Verification items for this drawing (mm, ordinates from the low corner). A direction names the side the tool comes from. Coordinates: 2 decimals unless noted, no trailing zeros. Order: outer loops, then holes, each group sorted by start corner. A loop starts at its lowest first (then second) coordinate and runs counter-clockwise, first axis right, second up. Notation, with made-up numbers: (-14, -26) - (30, -26) arc R25 cw to (30, -14) - close; hole circle Ø1 at (17, -10.5). An arc over 180 degrees is marked (long way). One line per question, with ' | ' between items. Start each with the question number.
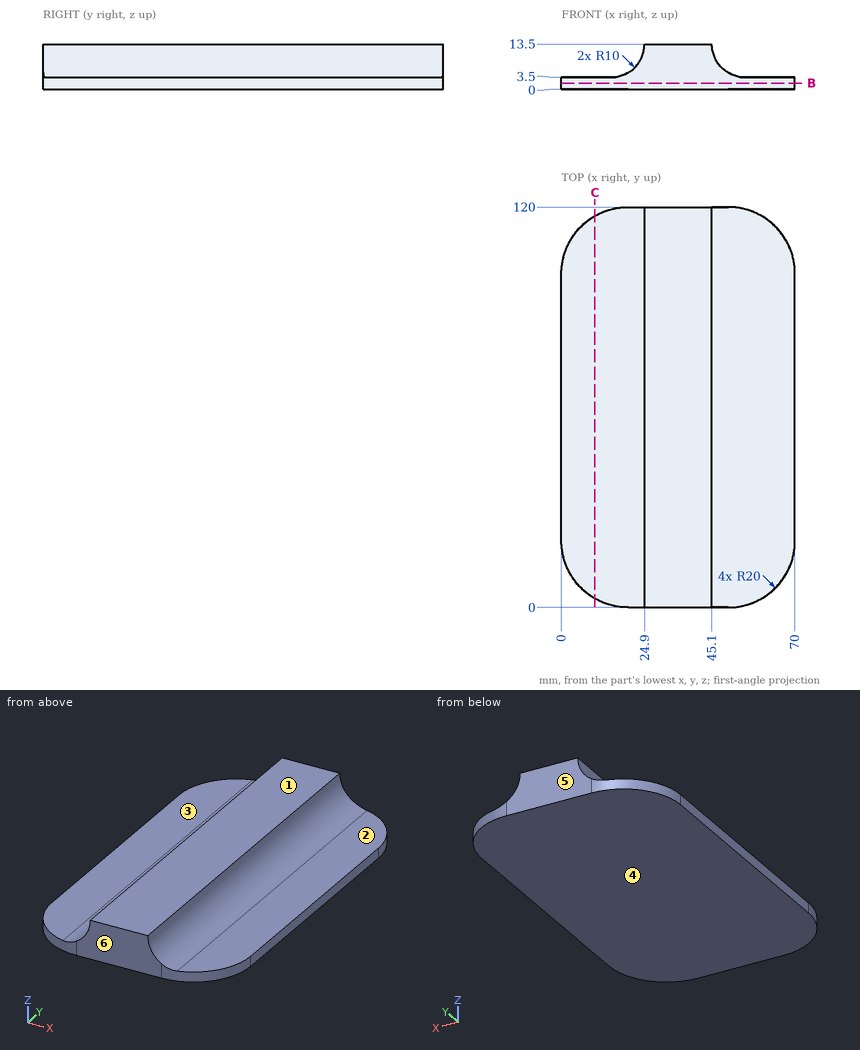
Item 1: Section check B-B (z = 1.75). Record the cut outline in (x, y).
Item 2: Gauge pin test, flat ends, axial feed: pin 1 (6 mm diameter, centred on x = 61.5, z = 6, fed in from -Y); pin 2 (5 mm diameter, centred on x = 62.5, z = 6.5, fed in from -Y); pin 3 (7.5 mm diameter, centred on x = 60, y = 49.5, fed in from +Z); pin 4 (8 mm diameter, centred on x = 16, y = 39, fed in from +Z). Record the tip position at first contact, or that the pin passes through.
Item 3: Section check C-C (x = 10). Record the cut outline in (y, z).
Item 4: Mould release check, pull along Y, two halves, no side actions. Record for the marked faces 4, 5 and 6: +Y half, -Y half, draft (parallel to the pull), parting line (faces both ways), or undercut.
Item 5: Set-up check for the marked faces 1, 2 and 3: record each of +Z, -Z, +X, -X, +Y, -Y from which the full face is reachable in a straight line by a thin tool's end or side.
Item 6: Thickness scan on probe 1 along Z at (x, y) = (66, 22); probe 2 along X at (y, z) = (24.5, 12.5); probe 3 along X at (y, z) = (58, 10.5). Record the ranges inside material, lowest first. Write a range as from..to.
Completed:
1) outline: (0, 20) arc R20 ccw to (20, 0) - (50, 0) arc R20 ccw to (70, 20) - (70, 100) arc R20 ccw to (50, 120) - (20, 120) arc R20 ccw to (0, 100) - close
2) pin 1: stops at y = 2.59 | pin 2: passes through | pin 3: stops at z = 3.5 | pin 4: stops at z = 4.9
3) outline: (2.68, 0) - (117.32, 0) - (117.32, 3.5) - (2.68, 3.5) - close
4) face 4: draft | face 5: +Y half | face 6: -Y half
5) face 1: +Z, +X, -X, +Y, -Y | face 2: +Z, +X, +Y, -Y | face 3: +Z, -X, +Y, -Y
6) probe 1: z = 0..3.5 | probe 2: x = 24.85..45.15 | probe 3: x = 24.44..45.56
